Could you check a few things on this model? Use its own coordinates, in mm. Face numbers are marked on the shaded views. A direction names the side the tool comes from. Give positions to 0.01 mm unless a question says otherwise; leave off trailing zeros. Order: outer loops, then holes, each group sorted by start corner. A loop starts at its lowest first (then second) coordinate and runs counter-clockwise, first axis right, second up. Notation, with made-up numbers: M -36.5,11.5 L 11.5,11.5 A26 ccw 11.5,45.5 Z; hole C -20,-35 d10. An arc over 180 degrees is marked long. Return JSON: item names as keys, results as strings. Group by question number.
```python
from build123d import *

# Parameters (mm, degrees)
SKETCH_1_W              = 5
SKETCH_1_H              = 20
EXTRUDE_1_DEPTH         = 5
SKETCH1_W               = 5
SKETCH1_H               = 20
EXTRUDE1_DEPTH          = 6.8
M2_5_TAPPED_HOLE1_D     = 2.05
M2_5_TAPPED_HOLE1_DEPTH = 6.35
M2_5_TAPPED_HOLE1_TIP   = 0.615882135
EXTRUDE2_DEPTH          = 2
CHAMFER1_SIZE           = 2
EXTRUDE3_START          = -5
SKETCH3_W               = 11.8
SKETCH3_H               = 3.5
EXTRUDE3_DEPTH          = 5
EXTRUDE4_DEPTH          = 2
CHAMFER2_SIZE           = 1
CHAMFER4_SIZE           = 3.5
CHAMFER4_SIZE2          = 6.062177826
SKETCH8_W               = 1
SKETCH8_H               = 16.5
EXTRUDE6_DEPTH          = 10
SKETCH11_W              = 5
SKETCH11_H              = 16.5
EXTRUDE8_DEPTH          = 0.5
EXTRUDE7_REACH          = 21.357
CHAMFER7_SIZE           = 1
FILLET1_R               = 5


with BuildPart() as part:
    # 草图1 → 拉伸1 (new body)
    with BuildSketch(Plane.XY):
        Rectangle(SKETCH_1_W, SKETCH_1_H)
    extrude(amount=EXTRUDE_1_DEPTH)

    # Sketch1 → Extrude1 (add)
    with BuildSketch(Plane.ZY.offset(2.5)):
        with Locations((2.5, 0)):
            Rectangle(SKETCH1_W, SKETCH1_H)
    extrude(amount=EXTRUDE1_DEPTH)

    # M2.5 Tapped Hole1
    with Locations(Plane(origin=(-1.5, -7, 5), x_dir=(1, 0, 0), z_dir=(0, 0, 1))):
        with Locations((0, 0), (-5.5, 5)):
            Hole(M2_5_TAPPED_HOLE1_D / 2, depth=M2_5_TAPPED_HOLE1_DEPTH)
            with Locations((0, 0, -(M2_5_TAPPED_HOLE1_DEPTH + M2_5_TAPPED_HOLE1_TIP / 2))):  # 118° drill point
                Cone(0, M2_5_TAPPED_HOLE1_D / 2, M2_5_TAPPED_HOLE1_TIP, mode=Mode.SUBTRACT)

    # Sketch2 → Extrude2 (cut)
    with BuildSketch(Plane(origin=(0, 0, 0), x_dir=(-1, 0, 0), z_dir=(0, 0, -1))):
        with BuildLine():
            Line((-2.383486142, -1.459806625), (0.079058889, 5.305980245))
            ThreePointArc((0.079058889, 5.305980245), (0.596133249, 5.870267889), (1.360771654, 5.903652722))
            Line((1.360771654, 5.903652722), (5.401449923, 4.432966106))
            ThreePointArc((5.401449923, 4.432966106), (5.965737567, 3.915891747), (5.9991224, 3.151253342))
            Line((5.9991224, 3.151253342), (3.536577368, -3.614533528))
            ThreePointArc((3.536577368, -3.614533528), (3.019503009, -4.178821171), (2.254864604, -4.212206005))
            Line((2.254864604, -4.212206005), (-1.785813665, -2.741519389))
            ThreePointArc((-1.785813665, -2.741519389), (-2.350101309, -2.22444503), (-2.383486142, -1.459806625))
        make_face()
    extrude(amount=-EXTRUDE2_DEPTH, mode=Mode.SUBTRACT)

    # Chamfer1
    chamfer1_edges = [part.edges().sort_by_distance(p)[0] for p in [
        (2.5, 0, 5),
    ]]
    chamfer(chamfer1_edges, length=CHAMFER1_SIZE)

    # Sketch3 → Extrude3 (cut)
    with BuildSketch(Plane.XY.offset(5).offset(EXTRUDE3_START)):
        with Locations((-3.4, 8.25)):
            Rectangle(SKETCH3_W, SKETCH3_H)
    extrude(amount=EXTRUDE3_DEPTH, mode=Mode.SUBTRACT)

    # Sketch4 → Extrude4 (cut)
    with BuildSketch(Plane(origin=(0, 0, 0), x_dir=(-1, 0, 0), z_dir=(0, 0, -1))):
        Polygon((-0.262961254, 4.366287624), (1.447139463, 9.064750728), (7.367202974, 6.910023825), (5.657102257, 2.211560721), align=None)
    extrude(amount=-EXTRUDE4_DEPTH, mode=Mode.SUBTRACT)

    # Chamfer2
    chamfer2_edges = [part.edges().sort_by_distance(p)[0] for p in [
        (-9.3, 6.5, 2.5),
    ]]
    chamfer(chamfer2_edges, length=CHAMFER2_SIZE)

    # Chamfer4
    chamfer4_edges = [part.edges().sort_by_distance(p)[0] for p in [
        (2.5, -10, 1.5),
    ]]
    chamfer4_side = [part.faces().sort_by_distance(p)[0] for p in [
        (-3.583625731, -10, 2.435672515),
    ]]
    chamfer(chamfer4_edges, length=CHAMFER4_SIZE, length2=CHAMFER4_SIZE2, reference=chamfer4_side[0])

    # Sketch8 → Extrude6 (cut)
    with BuildSketch(Plane.XY.offset(5)):
        with Locations((-8.8, -1.75)):
            Rectangle(SKETCH8_W, SKETCH8_H)
    extrude(amount=-EXTRUDE6_DEPTH, mode=Mode.SUBTRACT)

    # Sketch11 → Extrude8 (add)
    with BuildSketch(Plane.ZY.offset(8.3)):
        with Locations((2.5, -1.75)):
            Rectangle(SKETCH11_W, SKETCH11_H)
    extrude(amount=EXTRUDE8_DEPTH)

    # Extrude7: up to this face of the body (flat: up to its plane)
    extrude7_end = Plane(part.part.faces().sort_by_distance((-4.9, -10, 2.5))[0])
    # Sketch10 → Extrude7 (cut, up to the picked face)
    with BuildSketch(Plane(origin=(0, 6.5, 0), x_dir=(1, 0, 0), z_dir=(0, 1, 0)), mode=Mode.PRIVATE) as extrude7_sk1:
        Polygon((-8.8, -2), (-3.603847577, -5), (-8.8, -5), align=None)
    extrude7_tool1 = split(extrude(extrude7_sk1.sketch, amount=-EXTRUDE7_REACH, mode=Mode.PRIVATE), bisect_by=extrude7_end, keep=Keep.BOTH, mode=Mode.PRIVATE)
    add(extrude7_tool1.solids().sort_by(Axis((-7.067949, 6.5, 4), (0, -1, 0)))[0], mode=Mode.SUBTRACT)

    # Chamfer7
    chamfer7_edges = [part.edges().sort_by_distance(p)[0] for p in [
        (-8.8, -10, 1),
        (-8.8, 6.5, 1),
        (2.5, 6.5, 1.5),
    ]]
    chamfer(chamfer7_edges, length=CHAMFER7_SIZE)

    # Fillet1
    fillet1_edges = [part.edges().sort_by_distance(p)[0] for p in [
        (2.5, -3.937822174, 1.5),
    ]]
    fillet(fillet1_edges, radius=FILLET1_R)


solid = part.part
```
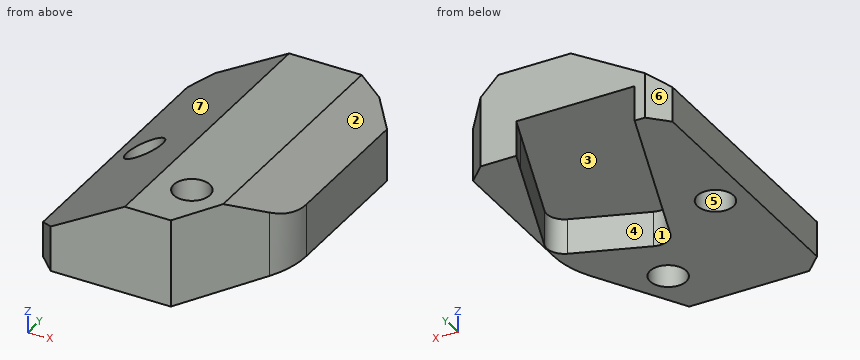
1. Which directions (+Z, -Z, +X, -X, +Y, -Y) give clear straight access to the entire face, cutting with the end or side of a thin tool? Please do the marked faces 1, 2 and 3.
2. Imagine slicing it at C-C, the plane y = -2. Please give me the cut outline in (x, z) (3 decimals).
3. If we mould it in two halves opening along Y, with no side actions, what happens to the marked faces 4, 5, 6 and 7? For each: pulls with the +Y half, pulls with the -Y half, needs draft (parallel to the pull), parting line crosses it, or undercut.
4. Imagine slicing it at B-B, the plane x = -7. Please give me the cut outline in (y, z) (3 decimals).
5. Imagine slicing it at D-D, the plane x = 1.25. Please give me the cut outline in (y, z).
6. For pin 1 (3 mm diameter, centred on y = 3.5, z = 4, fed in from +X), with a flat end and sliding along its axis, tell me the tip position at first contact or that it passes through.
7. I need wall thicknesses on L1, parallel to Y at x = -7, z = 2.45 (3 decimals); L2, parallel to Z at x = -3.25, y = 0.25; L3, parallel to Y at x = -1.5, z = 3.65 (3 decimals). Which ranges of each line are inside material? Lowest first, please. Write a range as from..to.
8. Imagine slicing it at A-A, the plane z = 1.3. Please give me the cut outline in (x, y) (3 decimals), plus the area to 3 significant figures.
Values:
{
 "1": {"face 1": "-Z, +Y", "face 2": "+Z, +X, +Y, -Y", "face 3": "-Z"},
 "2": {"outline": "M -8.8,0 L -8.025,0 L -8.025,2.447 L -8.8,2 Z; M -5.975,0 L -4.124,0 L -4.124,2 L 2.424,2 L 2.424,0 L 2.5,0 L 2.5,3 L 0.5,5 L -3.604,5 L -5.975,3.631 Z"},
 "3": {"face 4": "undercut", "face 5": "undercut", "face 6": "pulls with the +Y half", "face 7": "needs draft"},
 "4": {"outline": "M -10,0 L -3.025,0 L -3.025,3.039 L -10,3.039 Z; M -0.975,0 L 5.901,0 L 5.901,2 L 6.5,2 L 6.5,3.039 L -0.975,3.039 Z"},
 "5": {"outline": "M -6.1,0 L -2.94,0 L -2.94,2 L 1.65,2 L 1.65,0 L 6.5,0 L 6.5,4.25 L -6.1,4.25 Z"},
 "6": {"pin 1": "stops at x = 2.5"},
 "7": {"L1": "y = -10..-3.025, -0.975..6.5", "L2": "z = 2..5", "L3": "y = -10..-8.025, -5.975..6.5"},
 "8": {"outline": "M -8.8,-9 L -7.8,-10 L -1,-10 L 1.83,-5.098 A5 ccw 2.5,-2.598 L 2.5,5.5 L 1.5,6.5 L -0.514,6.5 L 2.383,-1.46 A1 cw 1.786,-2.742 L -2.255,-4.212 A1 cw -3.537,-3.615 L -7.218,6.5 L -7.8,6.5 L -8.8,5.5 Z; hole C -7,-2 d2.05; hole C -1.5,-7 d2.05", "area": "101 mm²"}
}
